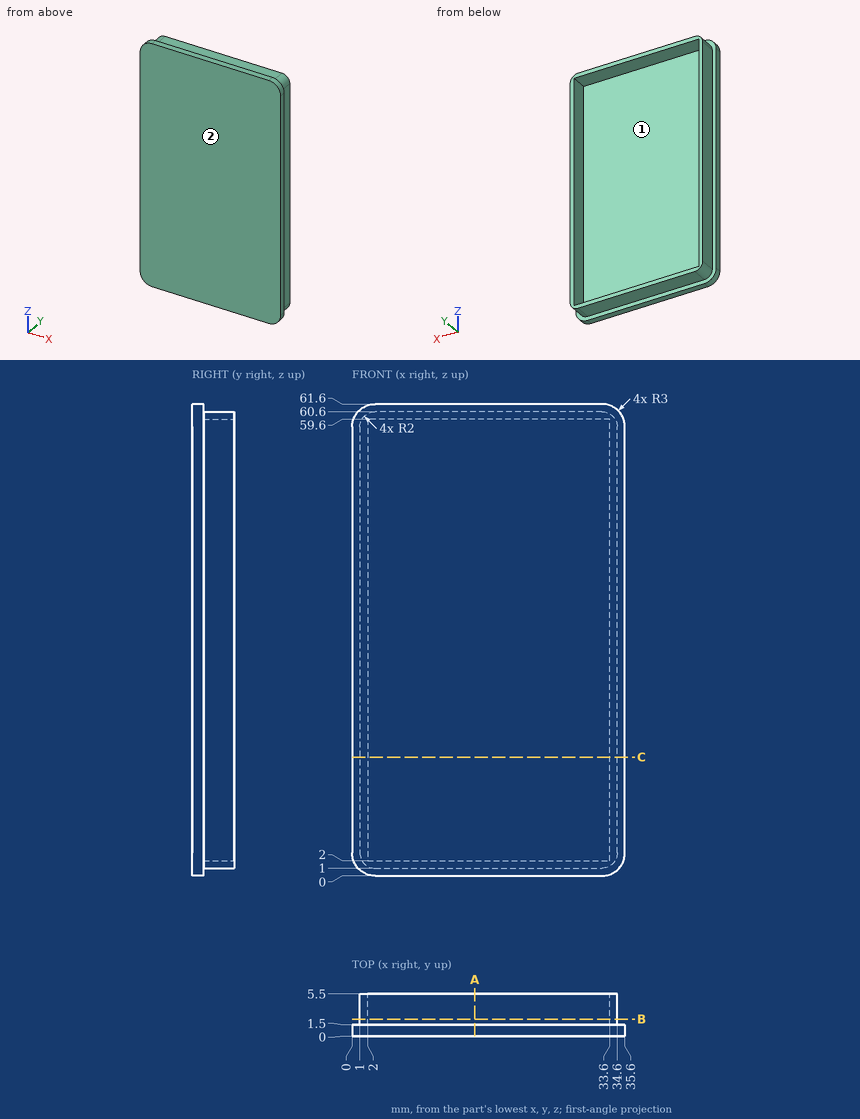
The figure shows three views and two pictorial views of one solid part (mm, origin at its lowest corner). Answer the questions. Give positions to 0.01 mm unless a question says otherwise; leave off trailing zeros. Write each loop counter-clockwise with the first axis right and the second up, starting at its lowest first coordinate (ties: lowest second). Pieces come first, ordered by that corner, then holes. Notation, with made-up numbers: (1, -31.75) - (46, -31.75) arc R14 ccw to (46, -7.75) - close; hole circle Ø2 at (-4.5, 16.25). An arc over 180 degrees is marked (long way). Use one line per item in the form item = value. Start each with the question number.
1) Find section B-B on y = 2.2. Determine the outline of the cut face in (x, z).
2) Find section A-A on x = 16. Determine the outline of the cut face in (y, z).
3) Find section C-C on z = 15.5. Determine the outline of the cut face in (x, y), plus the area to 3 significant figures.
4) Consider line 1 along X through (y, z) = (2.25, 58); line 2 along Z through (x, y) = (18, 5.05); line 3 along Y through (x, z) = (8, 13). Determine where each line is inside the solid, lowest interval first. Write a range as from..to.
5) Flat-ended cylindrical pins translate along their axes: pin 1 Ø2 at (x, y) = (16.5, 3.5) entering from -Z; pin 2 Ø2 at (y, z) = (4, 40) entering from -X; pin 3 Ø9.5 at (x, z) = (10.5, 21) entering from +Y. Find the tip coordinate at first contact, or state that the pin passes through.
6) The mould has two halves that part along X. Classify the marked faces 1 and 2: pulls with the +X half, pulls with the -X half, needs draft (parallel to the pull), parting line crosses it, or undercut.
Geometry results:
q1.outline = (1, 3) arc R2 ccw to (3, 1) - (32.6, 1) arc R2 ccw to (34.6, 3) - (34.6, 58.6) arc R2 ccw to (32.6, 60.6) - (3, 60.6) arc R2 ccw to (1, 58.6) - close; hole (2, 2) - (33.6, 2) - (33.6, 59.6) - (2, 59.6) - close
q2.outline = (0, 0) - (1.5, 0) - (1.5, 1) - (5.5, 1) - (5.5, 2) - (1.5, 2) - (1.5, 59.6) - (5.5, 59.6) - (5.5, 60.6) - (1.5, 60.6) - (1.5, 61.6) - (0, 61.6) - close
q3.outline = (0, 0) - (35.6, 0) - (35.6, 1.5) - (34.6, 1.5) - (34.6, 5.5) - (33.6, 5.5) - (33.6, 1.5) - (2, 1.5) - (2, 5.5) - (1, 5.5) - (1, 1.5) - (0, 1.5) - close
q3.area = 61.4 mm2
q4.line_1 = 1..2, 33.6..34.6
q4.line_2 = 1..2, 59.6..60.6
q4.line_3 = 0..1.5
q5.pin_1 = 1
q5.pin_2 = 1
q5.pin_3 = 1.5
q6.face_1 = undercut
q6.face_2 = needs draft
